Geometry: see drawing. Coordinates: mm, zero at the bounding-box minimum. Round coordinates to 2 decimals unless told otherwise and drop trailing zeros. Write each loop counter-clockwise with the first axis right and the second up, starting at its lowest first coordinate (ties: lowest second). Pieces come first, ordered by that corner, then holes.
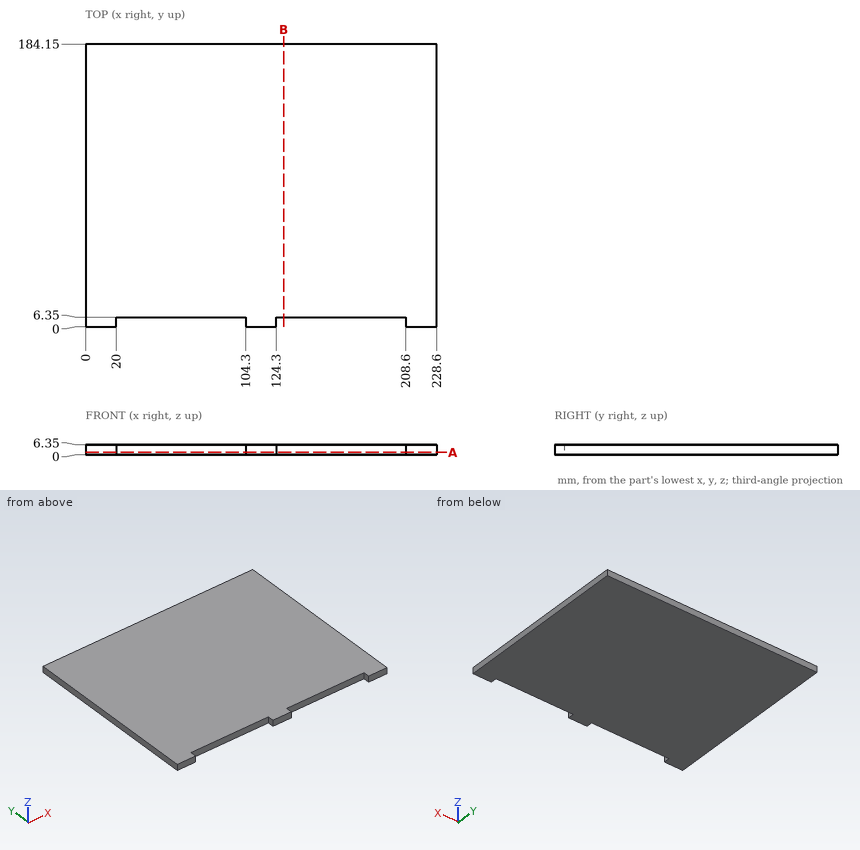
Q1. Section query A-A, the plane z = 1.5. Output: boundary loops of the cut face in (x, y).
Q2. Line query: line 1 (Y direction, x = 176, z = 3). Output: solid intervals per line, ascending.
Q3. Section query B-B, the plane x = 129. Output: boundary loops of the cut face in (y, z).
Q4. Pin query (flat end, axial travel): P1, Ø6, axis at x = 204, y = 152, coming from the -Z side; P2, Ø1.9, axis at x = 41.5, z = 2.5, coming from the -Y side. Return the tip coordinate at first contact, or that it passes through.
Filled in:
1. outline: (0, 0) - (20, 0) - (20, 6.35) - (104.3, 6.35) - (104.3, 0) - (124.3, 0) - (124.3, 6.35) - (208.6, 6.35) - (208.6, 0) - (228.6, 0) - (228.6, 184.15) - (0, 184.15) - close
2. line 1: y = 6.35 to 184.15
3. outline: (6.35, 0) - (184.15, 0) - (184.15, 6.35) - (6.35, 6.35) - close
4. P1: stops at z = 0
4. P2: stops at y = 6.35
